Autodesk Inventor part; units mm, degrees
ref_plane "YZ Plane" through (0, 0, 0) normal (1, 0, 0) x (0, 1, 0)
ref_plane "XZ Plane" through (0, 0, 0) normal (0, 1, 0) x (-1, 0, 0)
ref_plane "XY Plane" through (0, 0, 0) normal (0, 0, 1) x (1, 0, 0)
sketch "스케치1" plane through (0, 0, 0) normal (0, 1, 0) x (-1, 0, 0)
  line L0 (-55, 55) -> (55, 55)
  line L1 (55, 55) -> (55, -55)
  line L2 (55, -55) -> (-55, -55)
  line L3 (-55, -55) -> (-55, 55)
  line L4 (-55, 55) -> (55, -55) construction
  line L5 (55, 55) -> (-55, -55) construction
  point P0 (0, 0)
  dimension "d0" = 110
  dimension "d1" = 110
extrude "돌출1" add sketch "스케치1" along normal blind 5
fillet "모깎기1" radius 7 1 edges at (55, 2.5, 55)
fillet "모깎기2" radius 7 3 edges at (55, 2.5, -55) (-55, 2.5, -55) (-55, 2.5, 55)
sketch "스케치5" plane through (0, 0, 0) normal (0, -1, 0) x (1, 0, 0)
  arc A0 (55, 48) -> (48, 55) centre (48, 48) ccw
  circle A1 centre (48, 48) radius 3.5
  point P0 (0, 0)
  dimension "d15" = 7
extrude "돌출5" add sketch "스케치5" along normal blind 5
mirror "미러1" about plane through (0, 0, 0) normal (1, 0, 0) of "돌출5"
mirror "미러2" about plane through (0, 0, 0) normal (0, 0, 1) of "돌출5", "미러1"
sketch "스케치6" plane through (0, 5, 0) normal (0, 1, 0) x (1, 0, 0)
  arc A0 (-55, -48) -> (-48, -55) centre (-48, -48) ccw
  arc A1 (-48, 55) -> (-55, 48) centre (-48, 48) ccw
  arc A2 (55, 48) -> (48, 55) centre (48, 48) ccw
  arc A3 (48, -55) -> (55, -48) centre (48, -48) ccw
  circle A4 centre (-48, -48) radius 3.25
  point P0 (0, 0)
  dimension "d18" = 6.5
extrude "돌출6" cut sketch "스케치6" against normal blind 7
mirror "미러3" about plane through (0, 0, 0) normal (1, 0, 0) of "돌출6"
mirror "미러4" about plane through (0, 0, 0) normal (0, 0, 1) of "돌출6", "미러3"
sketch "스케치7" plane through (-48, -2, 48) normal (0, 1, 0) x (1, 0, 0)
  arc A0 (-7, 0) -> (0, -7) centre (0, 0) ccw
  circle A1 centre (0, 0) radius 1.8
  point P0 (48, 48)
  dimension "d21" = 3.6
extrude "돌출7" cut sketch "스케치7" against normal through all
mirror "미러5" about plane through (0, 0, 0) normal (0, 0, 1) of "돌출7"
mirror "미러6" about plane through (0, 0, 0) normal (1, 0, 0) of "돌출7", "미러5"
sketch "스케치9" plane through (0, 5, 0) normal (0, 1, 0) x (1, 0, 0)
  circle A0 centre (0, -15) radius 32.5
  line L0 (42.9638, 0) -> (-42.9638, 0) construction
  point P0 (0, 0)
  dimension "d32" = 65
  dimension "d33" = 15
extrude "돌출9" cut sketch "스케치9" against normal blind 1
sketch "스케치10" plane through (0, 4, 15) normal (0, 1, 0) x (1, 0, 0)
  circle A0 centre (0, 0) radius 22.5
  point P0 (0, 15)
  dimension "d36" = 45
extrude "돌출10" cut sketch "스케치10" against normal blind 1
sketch "스케치11" plane through (0, 3, 15) normal (0, 1, 0) x (1, 0, 0)
  circle A0 centre (0, 0) radius 19.5
  point P0 (0, 15)
  dimension "d39" = 39
extrude "돌출11" cut sketch "스케치11" against normal through all
chamfer "모따기2" distance 1 angle 45 1 edges at (-22.5, 4, 15)
sketch "스케치12" plane through (0, 4, 15) normal (0, 1, 0) x (1, 0, 0)
  circle A0 centre (0, 0) radius 26 construction
  circle A1 centre (0, -26) radius 2
  point P0 (0, 15)
  dimension "d48" = 52
  dimension "d49" = 4
extrude "돌출12" cut sketch "스케치12" against normal blind 10
pattern_circular "원형 패턴1" count 4 over 360 about axis through (0, 3.5, 15) along (0, 1, 0) of "돌출12"
properties part number "연결부"
Can you work these out from the model? Positions are in its coordinate system, mm. A direction names the side the tool comes from. Give positions to 0.01 mm unless a question says otherwise; leave off trailing zeros. Loops run counter-clockwise (first coordinate to the right, second up) from the corner with the lowest first, then second, coordinate; pieces in that order, holes last. Notation, with made-up numbers: (73, -22.5) - (132, -22.5) arc R28 cw to (132, 2.5) - close; hole circle Ø6 at (13.25, 48). An arc over 180 degrees is marked (long way). One line per item, written item: value.
(1) If we section it at A-A, the plane z = 15: State how many separate pieces and enclosed holes the cut face has, plus the area to 3 significant figures.
Verdict:
separate pieces: 4
enclosed holes: 0
area: 290 mm^2
(2) If we section it at B-B, the plane x = -26: List the corners of the cut face in (y, z) for me.
Verdict:
outline: (0, -55) - (5, -55) - (5, -4.5) - (4, -4.5) - (4, 13) - (0, 13) - close; (0, 17) - (4, 17) - (4, 34.5) - (5, 34.5) - (5, 55) - (0, 55) - close
(3) I'm going to push flat-ended pins straight in: pin 1 (5 mm diameter, centred on x = 26, z = 15, fed in from -Y); pin 2 (3.5 mm diameter, centred on x = -26, z = 15, fed in from -Y); pin 3 (2 mm diameter, centred on x = 49, z = -47.5, fed in from +Y); pin 4 (6.5 mm diameter, centred on x = 0, z = -11, fed in from +Y). Where does each tip first touch, or does it pass through?
Verdict:
pin 1: y = 0
pin 2: through
pin 3: y = -2
pin 4: y = 4
(4) If we section it at D-D, the plane z = -43: List the corners of the cut face in (x, y) for me, plus the area to 3 significant figures.
Verdict:
outline: (-55, 0) - (55, 0) - (55, 5) - (-55, 5) - close
area: 550 mm^2
(5) If we mould it in two halves opening along X, with no side actions, what happens to faces 4 (the face through (-27.2, 2, 13.4)), 5 (the face through (52.9, 2.5, 53)), 6 (the face through (28, 2, 15)), 7 (the face through (-55, 2, 1))? For each: released by +X, released by -X, zero draft, split by the parting line, or undercut.
Verdict:
face 4: undercut
face 5: released by +X
face 6: undercut
face 7: released by -X
(6) On a 3-axis mill with a long thin cutter (end or side, diameter ignored), from which of +Z, -Z, +X, -X, +Y, -Y can I reach the whole of each face in a straight line? I mean faces 1 (the face through (46.6, -2, -49.4)), 2 (the face through (-45.42, -2.465, -45.635)), 3 (the face through (48.234, -3.479, 49.785)). Say none if no direction works.
Verdict:
face 1: +Y
face 2: -Y
face 3: +Y, -Y
(7) If we section it at C-C, the plane z = -11: List the corners of the cut face in (x, y) for me, plus the area to 3 significant figures.
Verdict:
outline: (-55, 0) - (-2, 0) - (-2, 4) - (-19.5, 4) - (-19.5, 5) - (-55, 5) - close; (2, 0) - (55, 0) - (55, 5) - (19.5, 5) - (19.5, 4) - (2, 4) - close
area: 495 mm^2
(8) I need wall thicknesses on line 1 along X through (y, z) = (3.25, 48); line 2 along Z through (x, y) = (0, 4.5). Which ranges of each line are inside material? Lowest first, please.
Verdict:
line 1: -55 to -51.25, -44.75 to 44.75, 51.25 to 55
line 2: -55 to -17.5, 47.5 to 55
